The listing builds one solid part. Answer for the finished solid, in the listing's coordinates (mm). A direction names the side the tool comes from. Give positions to 0.01 mm unless a question says otherwise; leave off trailing zeros. Order: outer loops, then holes, each group sorted by start corner. A loop starts at its lowest first (then second) coordinate and runs counter-clockwise, first axis right, second up.
```python
from build123d import *

# Parameters (mm, degrees)
F0_W     = 100
F0_H     = 10
F1_DEPTH = 10
F2_W     = 8.5
F2_H     = 8.5
F3_DEPTH = 100
F4_R     = 2.871916
F5_DEPTH = 1


with BuildPart() as f1:
    # F0 (on Front) → F1 (new body)
    with BuildSketch(Plane.XZ):
        with Locations((-0.948794, -2.716295)):
            Rectangle(F0_W, F0_H)
    extrude(amount=F1_DEPTH)

    # F2 (on face) → F3 (join)
    with BuildSketch(Plane(origin=(-50.948794, 0, 0), x_dir=(0, -1, 0), z_dir=(-1, 0, 0))):
        with Locations((5, -2.716295)):
            Rectangle(F2_W, F2_H)
    extrude(amount=F3_DEPTH)

    # F4 (on face) → F5 (join)
    with BuildSketch(Plane.XZ.offset(10)):
        with Locations((19.08073, -2.832106)):
            Circle(F4_R)
    extrude(amount=F5_DEPTH)


solid = f1.part
```
1) Find section A-A (y = -5.75). Write down the section's boundary in (x, z), then the cut area to 3 significant figures.
Geometry says:
outline: (-150.95, -6.97) - (-50.95, -6.97) - (-50.95, -7.72) - (49.05, -7.72) - (49.05, 2.28) - (-50.95, 2.28) - (-50.95, 1.53) - (-150.95, 1.53) - close
area: 1,850 mm2
2) Find section B-B (x = -100.5). Write down the section's boundary in (y, z).
Geometry says:
outline: (-9.25, -6.97) - (-0.75, -6.97) - (-0.75, 1.53) - (-9.25, 1.53) - close
3) Find section C-C (x = -38). Write down the section's boundary in (y, z).
Geometry says:
outline: (-10, -7.72) - (0, -7.72) - (0, 2.28) - (-10, 2.28) - close
4) Straight lines are drawn through the part: probe 1 along Z at (x, y) = (-119, -4.5); probe 2 along Y at (x, z) = (-58, -5.75); probe 3 along X at (y, z) = (-9.5, -2.75). For each, find the intervals that lie inside material, in ascending order.
Geometry says:
probe 1: z = -6.97 to 1.53
probe 2: y = -9.25 to -0.75
probe 3: x = -50.95 to 49.05
5) Given P1, Ø1.5, axis at x = -100.5, y = -4.5, coming from the +Z side; P2, Ø5, axis at x = 1, z = -2, coming from the -Y side; P3, Ø4, axis at x = -117.5, z = -6, coming from the -Y side, each flat-ended and moving along its own axis, determine where each tip first touches the part or whether it passes through.
Geometry says:
P1: stops at z = 1.53
P2: stops at y = -10
P3: stops at y = -9.25
6) A tool of negligible diameter and unlimited length cuts with its end or side. For faces 1 (the flat face through (-100, -5, 1.534)), 2 (the flat face through (-100, -5, -6.966)), 3 (the cylindrical face through (16.21, -10.49, -2.71)), from which of +Z, -Z, +X, -X, +Y, -Y can it reach the whole face along a straight path? Write none if from no direction.
Geometry says:
face 1: +Z, -X, +Y, -Y
face 2: -Z, -X, +Y, -Y
face 3: -Y
